For this review, take the finished solid that the model builds, in its own axes (mm). Round coordinates to 2 decimals unless told otherwise and drop trailing zeros. Write each loop counter-clockwise with the first axis right and the second up, starting at its lowest first coordinate (ties: lowest second). Pieces come first, ordered by that corner, then holes. Notation, with made-up numbers: (33, 4) -> (58, 4) arc R29 ccw to (58, 32) -> close; hole circle Ø5 at (61.25, 54.5). An arc over 180 degrees is marked (long way). Answer in a Markdown table with one row per item. Add a question column.
```python
from build123d import *

# Parameters (mm, degrees)
F0_R     = 4.5
F1_DEPTH = 8
F4_R     = 1
F5_DEPTH = 12.501


with BuildPart() as f1:
    # F0 (on Front) → F1 (new body)
    with BuildSketch(Plane.XZ):
        Circle(F0_R)
    extrude(amount=F1_DEPTH)

    # F2 (on Right) → F3 (revolve)
    with BuildSketch(Plane.YZ):
        with BuildLine():
            Line((-8, 0), (-8, 4.5))
            ThreePointArc((-8, 4.5), (-11.181981, 3.181981), (-12.5, 0))
            Line((-12.5, 0), (-8, 0))
        make_face()
    revolve(axis=Axis((0, -26.326631, 0), (0, -1, 0)))

    # F4 (on Front) → F5 (cut, through all)
    with BuildSketch(Plane.XZ):
        Circle(F4_R)
    extrude(amount=F5_DEPTH, mode=Mode.SUBTRACT)


solid = f1.part
```
1. The part is to be moulded in two halves that separate along Z. For faces 1 (the cylindrical face through (0, -6, -1)), 2 (the flat face through (1, 0, -1)), 3 (the cylindrical face through (-0.59, -3.94, 4.46)), say which applies: pulls with the +Z half, pulls with the -Z half, needs draft (parallel to the pull), parting line crosses it, or undercut.
2. Clearance check with flat-ended pins moving along their axes: pin 1 Ø1.5 at (x, y) = (-3, -3.5) entering from -Z; pin 2 Ø3 at (x, z) = (-2, -3) entering from -Y. State where each tip first meets the part, or that it passes through.
3. We need section A-A (y = -0.75). Write out the cut boundary in (x, z), plus the area to 3 significant figures.
4. For L1, parallel to Z at x = 0, y = -6; L2, parallel to Z at x = -0.75, y = -8.75, list the stretches that pass through material, from the lowest coordinate up. Write a range as [from, to].
Response:
| question | item | result |
|---|---|---|
| 1 | face 1 | undercut |
| 1 | face 2 | needs draft |
| 1 | face 3 | parting line crosses it |
| 2 | pin 1 | z = -3.9 |
| 2 | pin 2 | y = -11.98 |
| 3 | outline | circle Ø9 at (0, 0); hole circle Ø2 at (0, 0) |
| 3 | area | 60.5 mm2 |
| 4 | L1 | [-4.5, -1], [1, 4.5] |
| 4 | L2 | [-4.37, -0.66], [0.66, 4.37] |
